For this review, take the finished solid that the model builds, in its own axes (mm). Give positions to 0.01 mm unless a question says otherwise; leave off trailing zeros. Loops run counter-clockwise (first coordinate to the right, second up) from the corner with the lowest first, then second, coordinate; pieces in that order, holes last. Notation, with made-up numbers: (-31.5, 85) - (-2.5, 85) arc R22 cw to (-2.5, 97) - close; hole circle Ø3 at (41.25, 37). An arc over 180 degrees is marked (long way). Answer as CSV lines item,"result".
from build123d import *

# Parameters (mm, degrees)
SKETCH1_R           = 8.5
BOSS_EXTRUDE1_DEPTH = 1
SKETCH2_R           = 8.5
SKETCH2_R_2         = 8
BOSS_EXTRUDE2_DEPTH = 25
CHAMFER1_SIZE       = 1


with BuildPart() as part:
    # Sketch1 → Boss-Extrude1 (new body)
    with BuildSketch(Plane.XY):
        Circle(SKETCH1_R)
    extrude(amount=BOSS_EXTRUDE1_DEPTH)

    # Sketch2 → Boss-Extrude2 (add)
    with BuildSketch(Plane.XY.offset(1)):
        Circle(SKETCH2_R)
        Circle(SKETCH2_R_2, mode=Mode.SUBTRACT)
    extrude(amount=BOSS_EXTRUDE2_DEPTH)

    # Chamfer1
    chamfer1_edges = [part.edges().sort_by_distance(p)[0] for p in [
        (-8, 0, 1),
    ]]
    chamfer(chamfer1_edges, length=CHAMFER1_SIZE)


solid = part.part
1) Consider section C-C on z = 17. Write out the cut boundary in (x, y), and give its area (3 significant figures).
From the geometry:
outline,"circle Ø17 at (0, 0); hole circle Ø16 at (0, 0)"
area,"25.9 mm^2"
2) Wall thickness on line 1 (Y direction, x = 0, z = 7.5); line 2 (Z direction, x = 5.75, y = 2.5): over which ranges is each line inside the solid? List them lowest first. Write a range as from..to.
From the geometry:
line 1,"y = -8.5..-8, 8..8.5"
line 2,"z = 0..1"
3) Consider section A-A on x = 0. Write out the cut boundary in (y, z).
From the geometry:
outline,"(-8.5, 0) - (8.5, 0) - (8.5, 26) - (8, 26) - (8, 2) - (7, 1) - (-7, 1) - (-8, 2) - (-8, 26) - (-8.5, 26) - close"
4) Draft analysis for pull direction X (two halves, no side actions). For faces 1 (the flat face through (0, 0, 0)), 2 (the flat face through (0, 0, 1)), 3 (the cylindrical face through (4.57, 7.167, 12.818)), state which applies: pulls with the +X half, pulls with the -X half, needs draft (parallel to the pull), parting line crosses it, or undercut.
From the geometry:
face 1,"needs draft"
face 2,"undercut"
face 3,"parting line crosses it"
5) Insertion check: P1, Ø1.5, axis at y = 2.5, z = 14.5, coming from the +X side; P2, Ø1, axis at y = -3, z = 4.5, coming from the +X side; P3, Ø6, axis at x = -2, y = 3, coming from the +Z side; P4, Ø6, axis at x = -2, y = -5.5, coming from the +Z side. Each pin has a flat end and moves straight along its axis. Give the tip position at first contact, or say it passes through.
From the geometry:
P1,"stops at x = 8.32"
P2,"stops at x = 8.12"
P3,"stops at z = 1"
P4,"stops at z = 26"
